```python
from build123d import *

# Parameters (mm, degrees)
FILLET1_R  = 25
FILLET12_R = 10


with BuildPart() as part:
    # Sketch1 → Revolve1 (revolve)
    with BuildSketch(Plane(origin=(0, 0, 0), x_dir=(0, 0, -1), z_dir=(1, 0, 0))):
        Polygon((0, 0), (5, 10.722534603), (5, 11.94189357), (25, 11.94189357), (25, 15.964993567), (5, 15.964993567), (5, 50), (0, 50), align=None)
    revolve(axis=Axis((0, 0, 0), (0, 1, 0)))

    # Fillet1
    # the kernel refuses this fillet: 25 mm, written as the material it adds along each edge
    with BuildSketch(Plane(origin=(0, 11.94189357, 0), x_dir=(0, 0, -1), z_dir=(1, 0, 0))) as fillet1_piece_1:
        with BuildLine():
            CenterArc((12.712399892, -25), FILLET1_R, 90, 17.968615565)
            Line((12.712399892, 0), (12.712399892, 0.5))
            Line((12.712399892, 0.5), (5, 0.5))
            Line((5, 0.5), (4.5, 0))
            ThreePointArc((4.5, 0), (4.5, -0.609679484), (4.845752002, -0.743746147))
            Line((4.845752002, -0.743746147), (5, -1.219358968))
        make_face()
    revolve(axis=Axis((0, 11.94189357, 0), (0, 1, 0)))

    # Fillet12
    fillet12_edges = [part.edges().sort_by_distance(p)[0] for p in [
        (0, 15.964993567, 5),
    ]]
    fillet(fillet12_edges, radius=FILLET12_R)


solid = part.part
```
Can you work these out from the model? Positions are in its coordinate system, mm. A direction names the side the tool comes from. Round coordinates to 2 decimals unless told otherwise and drop trailing zeros. Loops run counter-clockwise (first coordinate to the right, second up) from the corner with the lowest first, then second, coordinate; pieces in that order, holes last.
Item 1: Suppose I cut it at D-D, the plane y = 20. Write out the boundary of the cut face in (x, z).
Item 2: Suppose I cut it at B-B, the plane y = 38.5. Write out the boundary of the cut face in (x, z), then the cut area to 3 significant figures.
Item 3: Will these pins go through, and if not, where does the flat tip stop? pin 1 Ø12 at (x, y) = (-12.5, 17.5) entering from -Z; pin 2 Ø8 at (x, y) = (2, 40) entering from -Z; pin 3 Ø1.5 at (y, z) = (22.5, 0) entering from -X.
Item 4: Suppose I cut it at A-A, the plane x = -20. Write out the boundary of the cut face in (y, z) (3 decimals), then the cut area to 3 significant figures.
Item 5: Suppose I cut it at C-C, the plane z = -17. Write out the boundary of the cut face in (x, y) (3 decimals).
Item 6: Which directions (+Z, -Z, +X, -X, +Y, -Y) give clear straight access to the entire face, cutting with the end or side of a thin tool? Please do faces 1 (the flat face through (-5.9, 11.942, -11.5)), 2 (the flat face through (11, 15.965, -11)), 3 (the cylindrical face through (-7.509, 13.982, -23.846)).
Item 7: Please list where these lines run through material, in increasing order: L1, parallel to Y at x = -15, z = 8 (3 decimals); L2, parallel to Y at x = -8, z = -5; L3, parallel to Z at x = 8, y = 15.5.
Reported:
1. outline: circle Ø13.95 at (0, 0)
2. outline: circle Ø10 at (0, 0)
2. area: 78.5 mm2
3. pin 1: stops at z = -24.09
3. pin 2: stops at z = -5
3. pin 3: stops at x = -5.93
4. outline: (11.942, -15) - (15.965, -15) - (15.965, 15) - (11.942, 15) - close
4. area: 121 mm2
5. outline: (-18.33, 11.942) - (18.33, 11.942) - (18.33, 15.965) - (-18.33, 15.965) - close
6. face 1: -Y
6. face 2: +Y
6. face 3: +Y, -Y
7. L1: y = 11.942 to 15.965
7. L2: y = 11.73 to 17.66
7. L3: z = -23.69 to 23.69
